Here's how the part is built. I have some questions about the finished solid (model axes, mm). Round coordinates to 2 decimals unless told otherwise and drop trailing zeros. Loops run counter-clockwise (first coordinate to the right, second up) from the corner with the lowest first, then second, coordinate; pieces in that order, holes last. Notation, with made-up numbers: (-25, 6) -> (3, 6) arc R30 ccw to (3, 28) -> close; hole circle Ø5 at (89, 27.5). An arc over 180 degrees is marked (long way). One line per item, written item: value. Start each with the question number.
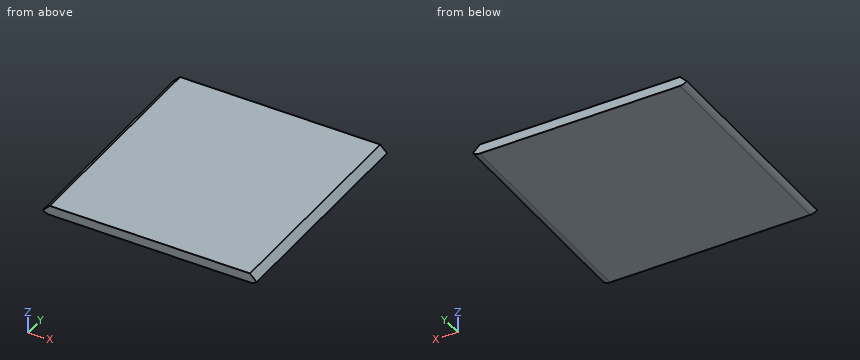
```python
from build123d import *

# Parameters (mm, degrees)
SKETCH1_W           = 105
SKETCH1_H           = 117
BOSS_EXTRUDE1_DEPTH = 5
BOSS_EXTRUDE2_DEPTH = 117


with BuildPart() as part:
    # Sketch1 → Boss-Extrude1 (new body)
    with BuildSketch(Plane.XY):
        Rectangle(SKETCH1_W, SKETCH1_H)
    extrude(amount=BOSS_EXTRUDE1_DEPTH)


with BuildPart() as body_2:
    # Sketch2 → Boss-Extrude2 (new body)
    with BuildSketch(Plane.XZ.offset(58.5)):
        with BuildLine():
            ThreePointArc((-52.5, 0), (-54.413417162, 0.380602337), (-56.035533906, 1.464466094))
            Line((-56.035533906, 1.464466094), (-52.5, 5))
            Line((-52.5, 5), (-52.5, 0))
        make_face()
    extrude(amount=-BOSS_EXTRUDE2_DEPTH)


with BuildPart() as body_3:
    # Mirror1: mirrored copy
    add(body_2.part.mirror(Plane.ZY))


with BuildPart() as body_2_1:
    add(body_2.part)

    # Combine1: union body 3, part
    add(body_3.part)
    add(part.part)


solid = body_2_1.part
```
Q1. I want a section at A-A on y = 38. Please give me the cut outline in (x, z), plus the area to 3 significant figures.
Q2. Will these pins go through, and if not, where does the flat tip stop? P1, Ø1.5, axis at y = -17, z = 3.5, coming from the -X side; P2, Ø1, axis at y = 4.5, z = 2.5, coming from the -X side.
Q3. I want a section at B-B on z = 4. Please give me the cut outline in (x, y).
Q4. If I drill on line 1 along X through (y, z) = (-1, 1.65); line 2 along X through (y, z) = (37.5, 3.55), over which ranges is the centre line in solid material (lowest first)?
Answers below:
1. outline: (-56.04, 1.46) arc R5 ccw to (-52.5, 0) -> (52.5, 0) arc R5 ccw to (56.04, 1.46) -> (52.5, 5) -> (-52.5, 5) -> close
1. area: 545 mm^2
2. P1: stops at x = -54.75
2. P2: stops at x = -55.5
3. outline: (-53.5, -58.5) -> (53.5, -58.5) -> (53.5, 58.5) -> (-53.5, 58.5) -> close
4. line 1: x = -55.85 to 55.85
4. line 2: x = -53.95 to 53.95
